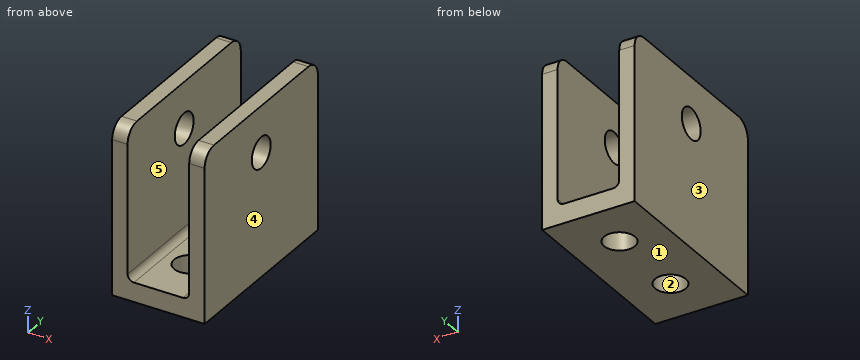
```python
from build123d import *

# Parameters (mm, degrees)
EXTRUDE1_DEPTH      = 19.05
SKETCH2_R           = 3.175
EXTRUDE2_DEPTH      = 35.925
SKETCH3_R           = 3.175
EXTRUDE3_DEPTH      = 10.525
EXTRUDE3_DEPTH_BACK = 10.525
FILLET3_R           = 3.1623
FILLET4_R           = 1.30175


with BuildPart() as part:
    # Sketch1 → Extrude1 (new body, symmetric)
    with BuildSketch(Plane(origin=(0, 0, 0), x_dir=(1, 0, 0), z_dir=(0, 1, 0))):
        Polygon((-9.525, 0), (9.525, 0), (9.525, -34.925), (6.35, -34.925), (6.35, -3.96875), (-6.35, -3.96875), (-6.35, -34.925), (-9.525, -34.925), align=None)
    extrude(amount=EXTRUDE1_DEPTH, both=True)

    # Sketch2 → Extrude2 (cut, through all)
    with BuildSketch(Plane.XY):
        with Locations((0, -8.5725)):
            Circle(SKETCH2_R)
        with Locations((0, 8.5725)):
            Circle(SKETCH2_R)
    extrude(amount=EXTRUDE2_DEPTH, mode=Mode.SUBTRACT)

    # Sketch3 → Extrude3 (cut, two sides)
    with BuildSketch(Plane(origin=(0, 0, -0.669808337), x_dir=(0, 0, -1), z_dir=(1, 0, 0))) as extrude3_sk:
        with Locations((-26.069808337, 0)):
            Circle(SKETCH3_R)
    extrude(amount=EXTRUDE3_DEPTH, mode=Mode.SUBTRACT)
    extrude(extrude3_sk.sketch, amount=-EXTRUDE3_DEPTH_BACK, mode=Mode.SUBTRACT)

    # Fillet3
    fillet3_edges = [part.edges().sort_by_distance(p)[0] for p in [
        (-7.9375, 19.05, 34.925),
        (7.9375, 19.05, 34.925),
        (7.9375, -19.05, 34.925),
        (-7.9375, -19.05, 34.925),
    ]]
    fillet(fillet3_edges, radius=FILLET3_R)

    # Fillet4
    fillet4_edges = [part.edges().sort_by_distance(p)[0] for p in [
        (6.35, 0, 3.96875),
        (-6.35, 0, 3.96875),
    ]]
    fillet(fillet4_edges, radius=FILLET4_R)


solid = part.part
```
The listing builds one solid part. Answer for the finished solid, in the listing's coordinates (mm). Face numbers are marked on the shaded views. A direction names the side the tool comes from. Give positions to 0.01 mm unless a question says otherwise; leave off trailing zeros. Order: outer loops, then holes, each group sorted by start corner. A loop starts at its lowest first (then second) coordinate and runs counter-clockwise, first axis right, second up. Notation, with made-up numbers: (-4.5, 88.25) - (38.5, 88.25) arc R21 ccw to (38.5, 123.25) - close; hole circle Ø4 at (-33, -27.5). An arc over 180 degrees is marked (long way). Answer in a Markdown table with one row per item. Add a question column.
Q1. Find the intervals of material crossed by line 1 along Y through (x, z) = (0, 1.5); line 2 along Y through (x, z) = (-8.2, 25.4) (3 decimals); line 3 along X through (y, z) = (-15, 12) (3 decimals), in increasing order. Write a range as [from, to].
Q2. Given P1, Ø4, axis at x = 0, y = 8.57, coming from the +Z side; P2, Ø10, axis at x = 0, y = -8.57, coming from the +Z side; P3, Ø11, axis at x = -0.5, y = 8.5, coming from the +Z side, each flat-ended and moving along its own axis, determine where each tip first touches the part or whether it passes through.
Q3. The part is cut by section D-D (x = 0). Determine the outline of the cut face in (y, z), then the cut area to 3 significant figures.
Q4. The part is cut by section A-A (z = 17). Determine the outline of the cut face in (x, y) (3 decimals), then the cut area to 3 significant figures.
Q5. The part is cut by section C-C (z = 25.4). Determine the outline of the cut face in (x, y) (3 decimals).
Q6. Which of the six approach directions +Z, -Z, +X, -X, +Y, -Y give full straight-line access (tool end or side, diameter ignored) to the marked faces 4 and 5?
Q7. The part is cut by section B-B (y = 0). Give the number of separate pieces and of enclosed holes in the cut face, then the cut area to 3 significant figures.
Q8. For a pull along X with two mould halves and no side action, classify the marked faces 1, 2 and 3 as released by +X, released by -X, zero draft, split by the parting line, or undercut.
Determined:
| question | item | result |
|---|---|---|
| 1 | line 1 | y = [-19.05, -11.75], [-5.4, 5.4], [11.75, 19.05] |
| 1 | line 2 | y = [-19.05, -3.175], [3.175, 19.05] |
| 1 | line 3 | x = [-9.525, -6.35], [6.35, 9.525] |
| 2 | P1 | passes through |
| 2 | P2 | stops at z = 3.97 |
| 2 | P3 | stops at z = 4.38 |
| 3 | outline | (-19.05, 0) - (-11.75, 0) - (-11.75, 3.97) - (-19.05, 3.97) - close; (-5.4, 0) - (5.4, 0) - (5.4, 3.97) - (-5.4, 3.97) - close; (11.75, 0) - (19.05, 0) - (19.05, 3.97) - (11.75, 3.97) - close |
| 3 | area | 101 mm² |
| 4 | outline | (-9.525, -19.05) - (-6.35, -19.05) - (-6.35, 19.05) - (-9.525, 19.05) - close; (6.35, -19.05) - (9.525, -19.05) - (9.525, 19.05) - (6.35, 19.05) - close |
| 4 | area | 242 mm² |
| 5 | outline | (-9.525, -19.05) - (-6.35, -19.05) - (-6.35, -3.175) - (-9.525, -3.175) - close; (-9.525, 3.175) - (-6.35, 3.175) - (-6.35, 19.05) - (-9.525, 19.05) - close; (6.35, -19.05) - (9.525, -19.05) - (9.525, -3.175) - (6.35, -3.175) - close; (6.35, 3.175) - (9.525, 3.175) - (9.525, 19.05) - (6.35, 19.05) - close |
| 6 | face 4 | +Z, -Z, +X, +Y, -Y |
| 6 | face 5 | +Z, +Y, -Y |
| 7 | separate pieces | 3 |
| 7 | enclosed holes | 0 |
| 7 | area | 233 mm² |
| 8 | face 1 | zero draft |
| 8 | face 2 | undercut |
| 8 | face 3 | released by -X |
